Geometry: final body of the model. Coordinates: model frame, mm. A direction names the side the tool comes from. Give positions to 0.01 mm unless a question says otherwise; leave off trailing zeros. Write each loop counter-clockwise with the first axis right and the second up, starting at its lowest first coordinate (ties: lowest second). Pieces come first, ordered by that corner, then holes. Notation, with made-up numbers: (-13.75, -14.5) - (27.25, -14.5) arc R26 ccw to (27.25, 6.5) - close; hole circle Ø10 at (-3.5, -6.5). An arc over 180 degrees is marked (long way). Return JSON: item names as keys, results as strings.
from build123d import *

# Parameters (mm, degrees)
CROQUIS1_R              = 1.000000138
CROQUIS1_R_2            = 0.999999989
SALIENTE_EXTRUIR1_DEPTH = 3
SALIENTE_EXTRUIR2_DEPTH = 3.25
CROQUIS3_W              = 5.000000382
CROQUIS3_H              = 25
CROQUIS3_W_2            = 5.000000381
SALIENTE_EXTRUIR3_DEPTH = 5.75
CROQUIS4_R              = 1
CORTAR_EXTRUIR1_DEPTH   = 11.35
CROQUIS5_R              = 1
CORTAR_EXTRUIR2_DEPTH   = 11.35
CROQUIS6_R              = 1.000000138
CROQUIS6_R_2            = 0.999999989
CORTAR_EXTRUIR3_DEPTH   = 11.35


with BuildPart() as part:
    # Croquis1 → Saliente-Extruir1 (new body)
    with BuildSketch(Plane(origin=(0, 0, 0), x_dir=(1, 0, 0), z_dir=(0, 1, 0))):
        with BuildLine():
            Line((7.826252673, -7.136543799), (16.57691182, -7.136543799))
            Line((16.57691182, -7.136543799), (16.57691182, 17.863456201))
            Line((16.57691182, 17.863456201), (-16.123088943, 17.863456201))
            Line((-16.123088943, 17.863456201), (-16.123088943, -7.136543799))
            Line((-16.123088943, -7.136543799), (-7.372430407, -7.136543799))
            ThreePointArc((-7.372430407, -7.136543799), (0.226911133, -17.636544763), (7.826252673, -7.136543799))
        make_face()
        with Locations((0.226911587, 13.863456348)):
            Circle(CROQUIS1_R, mode=Mode.SUBTRACT)
        with Locations((0.226910898, -14.136544906)):
            Circle(CROQUIS1_R_2, mode=Mode.SUBTRACT)
        with BuildLine():
            ThreePointArc((-3.120375102, 0.386039479), (0.227925042, -4.136543652), (3.573605207, 0.387978009))
            ThreePointArc((3.573605207, 0.387978009), (0.223436552, 11.362755325), (-3.120375102, 0.386039479))
        make_face(mode=Mode.SUBTRACT)
    extrude(amount=SALIENTE_EXTRUIR1_DEPTH)

    # Croquis2 → Saliente-Extruir2 (add)
    with BuildSketch(Plane(origin=(0, 3, 0), x_dir=(1, 0, 0), z_dir=(0, 1, 0))):
        with BuildLine():
            Line((-7.519055395, -11.636544922), (7.972877662, -11.636544922))
            ThreePointArc((7.972877662, -11.636544922), (0.226911133, -17.636544763), (-7.519055395, -11.636544922))
        make_face()
        Polygon((-16.123088943, 17.863456201), (-11.123088561, 17.863456201), (-11.123088561, 16.363456201), (11.576911439, 16.363456201), (11.576911439, 17.863456201), (16.57691182, 17.863456201), (16.57691182, -7.136543799), (8.226911439, -7.136543799), (8.226911439, -4.636543799), (11.576911439, -4.636543799), (11.576911439, 11.362755577), (-11.123088561, 11.362755577), (-11.123088561, -4.636543799), (-7.773088561, -4.636543799), (-7.773088561, -7.136543799), (-16.123088943, -7.136543799), align=None)
    extrude(amount=SALIENTE_EXTRUIR2_DEPTH)

    # Croquis3 → Saliente-Extruir3 (add)
    with BuildSketch(Plane(origin=(0, 6.25, 0), x_dir=(1, 0, 0), z_dir=(0, 1, 0))):
        with Locations((-13.623088752, 5.363456201)):
            Rectangle(CROQUIS3_W, CROQUIS3_H)
        with Locations((14.076911629, 5.363456201)):
            Rectangle(CROQUIS3_W_2, CROQUIS3_H)
    extrude(amount=SALIENTE_EXTRUIR3_DEPTH)

    # Croquis4 → Cortar-Extruir1 (cut)
    with BuildSketch(Plane.ZY.offset(16.123088943)):
        with Locations((-11.363456201, 6)):
            Circle(CROQUIS4_R)
        with Locations((0.636543799, 6)):
            Circle(CROQUIS4_R)
    extrude(amount=-CORTAR_EXTRUIR1_DEPTH, mode=Mode.SUBTRACT)

    # Croquis5 → Cortar-Extruir2 (cut)
    with BuildSketch(Plane(origin=(16.57691182, 0, 0), x_dir=(0, 0, -1), z_dir=(1, 0, 0))):
        with Locations((11.363456201, 6)):
            Circle(CROQUIS5_R)
        with Locations((-0.636543799, 6)):
            Circle(CROQUIS5_R)
    extrude(amount=-CORTAR_EXTRUIR2_DEPTH, mode=Mode.SUBTRACT)

    # Croquis6 → Cortar-Extruir3 (cut)
    with BuildSketch(Plane.XZ):
        with Locations((0.226911587, -13.863456348)):
            Circle(CROQUIS6_R)
        with Locations((0.226910898, 14.136544906)):
            Circle(CROQUIS6_R_2)
    extrude(amount=-CORTAR_EXTRUIR3_DEPTH, mode=Mode.SUBTRACT)


solid = part.part
Q1. Pin query (flat end, axial travel): P1, Ø2.5, axis at x = 0.23, z = -13.86, coming from the -Y side; P2, Ø1.6, axis at x = 0.23, z = -13.86, coming from the +Y side; P3, Ø1.8, axis at x = -2, z = 13.5, coming from the +Y side; P4, Ø4, axis at x = -8, z = -6.5, coming from the +Y side. Return the tip coordinate at first contact, or that it passes through.
Answer key:
{"P1": "stops at y = 0", "P2": "passes through", "P3": "stops at y = 6.25", "P4": "stops at y = 3"}
Q2. Section query D-D, the plane x = -1.5. Return the cut outline in (y, z).
Answer key:
{"outline": "(0, -17.86) - (3, -17.86) - (3, -16.36) - (6.25, -16.36) - (6.25, -11.36) - (3, -11.36) - (3, -11.11) - (0, -11.11) - close; (0, 3.68) - (3, 3.68) - (3, 11.64) - (6.25, 11.64) - (6.25, 17.45) - (0, 17.45) - close"}
Q3. Set-up query: faces 1 (the flat face through (0, 4, -11.363)), 2 (the flat face through (10, 6.25, 6)), 3 (the flat face through (0, 5, 11.637)). Return all of +Z, -Z, +X, -X, +Y, -Y with unobstructed straight access to the full face (end or side cutting, diameter ignored); none if empty.
Answer key:
{"face 1": "+Y", "face 2": "+Z, -Z, +Y", "face 3": "+X, -X, +Y"}
Q4. Material intervals for probe 1 along X at (y, z) = (4, -0.5); probe 2 along Z at (x, y) = (13, 6.25); probe 3 along Z at (x, y) = (0.5, 3.75), sorted ascending. Write a range as [from, to].
Answer key:
{"probe 1": "x = [-16.12, -11.12], [11.58, 16.58]", "probe 2": "z = [-17.86, -12.33], [-10.4, -0.33], [1.6, 7.14]", "probe 3": "z = [-16.36, -14.83], [-12.9, -11.36], [11.64, 13.17], [15.1, 17.63]"}
Q5. Mould query, pull axis X, two halves, no side actions, for faces 4 (the flat face through (5.227, 6, -12)), 5 (the flat face through (4, 0, 0)), 6 (the flat face through (-9, 5, 4.637)). Classes: pulls with the +X half, pulls with the -X half, needs draft (parallel to the pull), parting line crosses it, or undercut.
Answer key:
{"face 4": "pulls with the +X half", "face 5": "needs draft", "face 6": "undercut"}
Q6. Section query C-C, the plane z = -5. Return the cut outline in (x, y).
Answer key:
{"outline": "(-16.12, 0) - (-5.76, 0) - (-5.76, 3) - (-11.12, 3) - (-11.12, 12) - (-16.12, 12) - close; (6.21, 0) - (16.58, 0) - (16.58, 12) - (11.58, 12) - (11.58, 3) - (6.21, 3) - close"}
Q7. Section query B-B, the plane y = 3.75. Return the cut outline in (x, z), plus the area to 3 significant figures.
Answer key:
{"outline": "(-16.12, -17.86) - (-11.12, -17.86) - (-11.12, -16.36) - (11.58, -16.36) - (11.58, -17.86) - (16.58, -17.86) - (16.58, 7.14) - (8.23, 7.14) - (8.23, 4.64) - (11.58, 4.64) - (11.58, -11.36) - (-11.12, -11.36) - (-11.12, 4.64) - (-7.77, 4.64) - (-7.77, 7.14) - (-16.12, 7.14) - close; (-7.52, 11.64) - (7.97, 11.64) arc R8 ccw to start; hole circle Ø2 at (0.23, -13.86); hole circle Ø2 at (0.23, 14.14)", "area": "443 mm^2"}
Q8. Section query A-A, the plane y = 8.25. Return the cut outline in (x, z), plus the area to 3 significant figures.
Answer key:
{"outline": "(-16.12, -17.86) - (-11.12, -17.86) - (-11.12, 7.14) - (-16.12, 7.14) - close; (11.58, -17.86) - (16.58, -17.86) - (16.58, 7.14) - (11.58, 7.14) - close", "area": "250 mm^2"}
